Could you check a few things on this model? Use its own coordinates, in mm. Face numbers are marked on the shaded views. Round coordinates to 2 decimals unless told otherwise and drop trailing zeros. Loops run counter-clockwise (first coordinate to the right, second up) from the corner with the lowest first, then second, coordinate; pieces in that order, holes last.
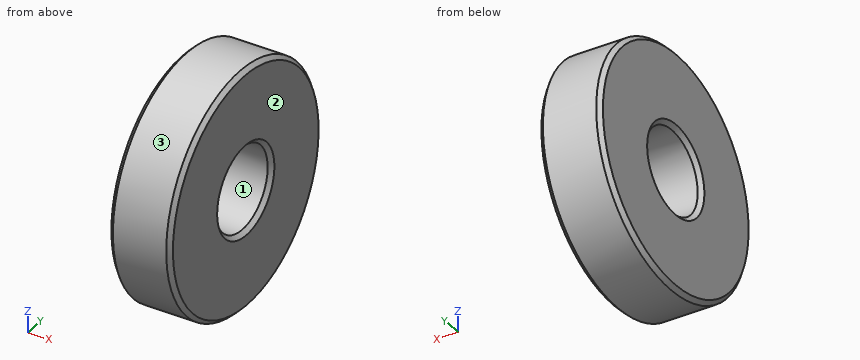
from build123d import *

# Parameters (mm, degrees)
CROQUIS1_R              = 2.9
CROQUIS1_R_2            = 1
SALIENTE_EXTRUIR1_DEPTH = 1.5
CHAFL_N1_SIZE           = 0.1


with BuildPart() as part:
    # Croquis1 → Saliente-Extruir1 (new body)
    with BuildSketch(Plane(origin=(0, 0, 0), x_dir=(0, 0, -1), z_dir=(1, 0, 0))):
        Circle(CROQUIS1_R)
        Circle(CROQUIS1_R_2, mode=Mode.SUBTRACT)
    extrude(amount=SALIENTE_EXTRUIR1_DEPTH)

    # Chaflán1
    chafl_n1_edges = [part.edges().sort_by_distance(p)[0] for p in [
        (0, 0, 2.9),
        (1.5, 0, 2.9),
        (0, 0, 1),
        (1.5, 0, 1),
    ]]
    chamfer(chafl_n1_edges, length=CHAFL_N1_SIZE)


solid = part.part
Item 1: If we section it at A-A, the plane z = 0: Please give me the cut outline in (x, y).
Results list:
outline: (0, -2.8) - (0.1, -2.9) - (1.4, -2.9) - (1.5, -2.8) - (1.5, -1.1) - (1.4, -1) - (0.1, -1) - (0, -1.1) - close; (0, 1.1) - (0.1, 1) - (1.4, 1) - (1.5, 1.1) - (1.5, 2.8) - (1.4, 2.9) - (0.1, 2.9) - (0, 2.8) - close
Item 2: If we section it at C-C, the plane x = 1.15: Please give me the cut outline in (y, z).
Results list:
outline: circle Ø5.8 at (0, 0); hole circle Ø2 at (0, 0)
Item 3: We'd pull the mould along Y, two halves only. Please class the marked faces 1, 2 and 3: released by +Y, released by -Y, zero draft, split by the parting line, or undercut.
Results list:
face 1: undercut
face 2: zero draft
face 3: split by the parting line
Item 4: If I drill on line 1 along Y through (x, z) = (1.05, 0); line 2 along Y through (x, z) = (0.9, -0.55); line 3 along Y through (x, z) = (0.45, -1.8), over which ranges is the centre line in solid material (lowest first)?
Results list:
line 1: y = -2.9 to -1, 1 to 2.9
line 2: y = -2.85 to -0.84, 0.84 to 2.85
line 3: y = -2.27 to 2.27
